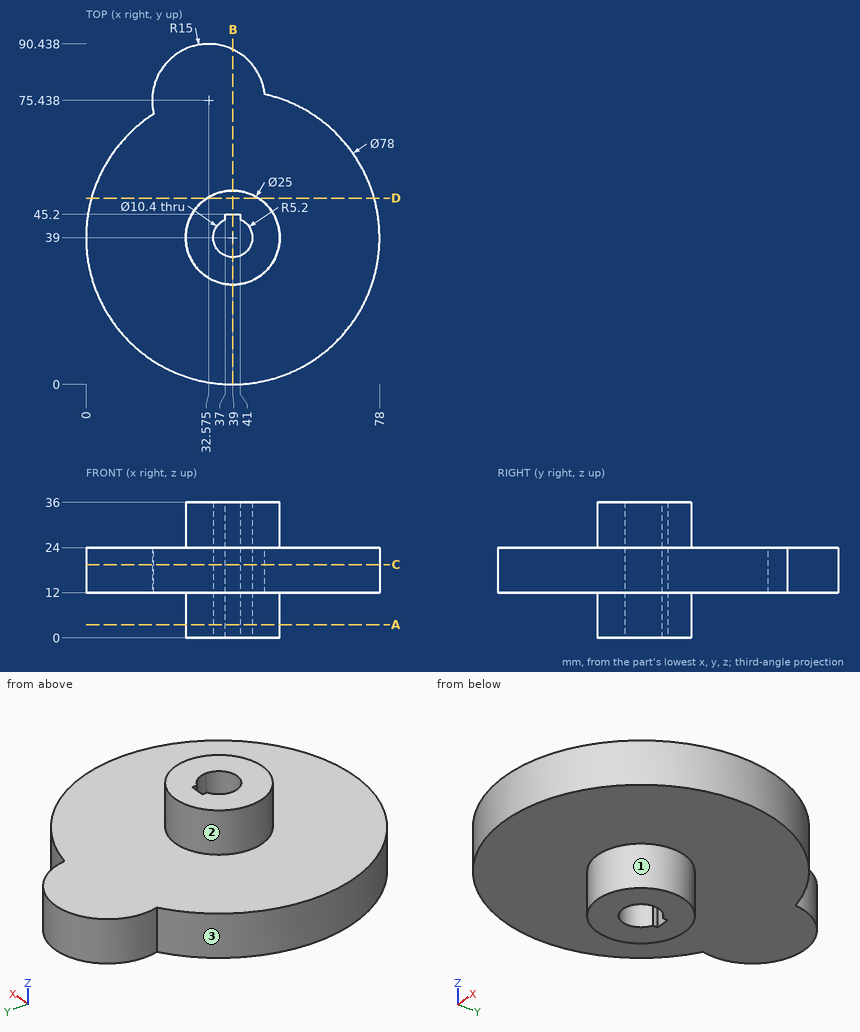
Part print with two shaded views. Sizes in mm from the minimum x, y, z corner. A direction names the side the tool comes from. Give positions to 0.01 mm unless a question says otherwise; leave off trailing zeros. Order: outer loops, then holes, each group sorted by start corner. A loop starts at its lowest first (then second) coordinate and runs counter-clockwise, first axis right, second up.
(1) Saw through at C-C, the plane z = 19.5. Give the cut face in (x, y) (1 decimal).
(2) Tool access for the marked faces 1, 2 and 3: list every direction of +Z, -Z, +X, -X, +Y, -Y with a clear straight run to the whole face (end or side of a thin tool).
(3) Saw through at D-D, the plane y = 49.5. Give the cut face in (x, z).
(4) Flat gauge pins, fed straight in: pin 1 (10 mm diameter, centred on y = 71, z = 20, fed in from +X); pin 2 (1.5 mm diameter, centred on x = 21, y = 48, fed in from -Z); pin 3 (12 mm diameter, centred on x = 39, y = 39, fed in from -Z); pin 4 (0.7 mm diameter, centred on y = 44.5, z = 15, fed in from -X). Where does each tip first touch, or does it go through?
(5) Saw through at B-B, the plane x = 39. Give the cut face in (y, z).
(6) Drill centre lines: L1, parallel to Y at x = 39, z = 26; L2, parallel to X at y = 39, z = 11; L3, parallel to Z at x = 57, y = 18. Where is each one in solid material? Low to high.
(7) Saw through at A-A, the plane z = 3.5. Give the cut face in (x, y), then the cut area to 3 significant figures.
Results found:
1. outline: (18, 71.9) arc R39 ccw (long way) to (47.5, 77.1) arc R15 ccw (long way) to start; hole (37, 43.8) arc R5.2 ccw (long way) to (41, 43.8) - (41, 45.2) - (37, 45.2) - close
2. face 1: -Z
2. face 2: +Z
2. face 3: +Z, -Z
3. outline: (1.44, 12) - (32.22, 12) - (32.22, 0) - (45.78, 0) - (45.78, 12) - (76.56, 12) - (76.56, 24) - (45.78, 24) - (45.78, 36) - (32.22, 36) - (32.22, 24) - (1.44, 24) - close
4. pin 1: stops at x = 67.14
4. pin 2: stops at z = 12
4. pin 3: stops at z = 0
4. pin 4: stops at x = 0.34
5. outline: (0, 12) - (26.5, 12) - (26.5, 0) - (33.8, 0) - (33.8, 36) - (26.5, 36) - (26.5, 24) - (0, 24) - close; (45.2, 0) - (51.5, 0) - (51.5, 12) - (88.99, 12) - (88.99, 24) - (51.5, 24) - (51.5, 36) - (45.2, 36) - close
6. L1: y = 26.5 to 33.8, 45.2 to 51.5
6. L2: x = 26.5 to 33.8, 44.2 to 51.5
6. L3: z = 12 to 24
7. outline: circle Ø25 at (39, 39); hole (37, 43.8) arc R5.2 ccw (long way) to (41, 43.8) - (41, 45.2) - (37, 45.2) - close
7. area: 401 mm2
